Geometry check sheet. Reference: the model listing, model coordinates, mm. A direction names the side the tool comes from. Round coordinates to 2 decimals unless told otherwise and drop trailing zeros. Order: outer loops, then holes, each group sorted by start corner. A loop starts at its lowest first (then second) coordinate and runs counter-clockwise, first axis right, second up. Notation, with made-up numbers: (41, -25) -> (69, -25) arc R21 ccw to (69, 2) -> close; hole circle Ø8 at (-28.75, 2). An arc over 180 degrees is marked (long way). Use a Markdown table: item, result. Add a question column.
Item 1: Sectioned sample at A-A, the plane z = 13. Record the cut outline in (x, y).
Item 2: Sectioned sample at C-C, the plane y = 14.25. Record the cut outline in (x, z).
Item 3: Set-up check for faces 4 (the cylindrical face through (-18.66, 12.96, 23.61)), 5 (the flat face through (26.289, 10, 0)), 6 (the cylindrical face through (-4.69, 2.5, -3.59)): record each of +Z, -Z, +X, -X, +Y, -Y from which the full face is reachable in a straight line by a thin tool's end or side.
Item 4: Gauge pin test, flat ends, axial feed: pin 1 Ø6 at (x, z) = (6, 8.5) entering from +Y; pin 2 Ø6 at (x, z) = (17.907, -17.907) entering from +Y; pin 3 Ø15.5 at (x, z) = (0, 0) entering from +Y. Record the tip position at first contact, or that the pin passes through.
Item 5: Mould release check, pull along Z, two halves, no side actions. Record for faces 1 (the flat face through (0, 10, -26.289)), 2 (the flat face through (-0.4, 0, -6.2)), 3 (the cylindrical face through (15.94, 2.84, -19.71)): pulls with the +Z half, pulls with the -Z half, needs draft (parallel to the pull), parting line crosses it, or undercut.
Item 6: Material ranges on probe 1 along Z at (x, y) = (0, 3.45); probe 2 along Z at (x, y) = (-18, 16); probe 3 along Z at (x, y) = (0, 8.75), recorded low to high. Write a range as [from, to].
Item 7: Sectioned sample at B-B, the plane x = -16. Record the cut outline in (y, z), and give its area (3 significant figures).
Item 8: Sectioned sample at D-D, the plane y = 10.25. Record the cut outline in (x, z).
from build123d import *

# Parameters (mm, degrees)
SKETCH1_W       = 52.578
SKETCH1_H       = 52.578
EXTRUDE1_DEPTH  = 19.9644
EXTRUDE2_START  = -19.9644
SKETCH2_R       = 2.667
EXTRUDE2_DEPTH  = 5.7658
EXTRUDE4_START  = -19.9644
SKETCH6_R       = 5.75437
EXTRUDE4_DEPTH  = 14.1986
EXTRUDE6_START  = -45.52216
EXTRUDE6_DEPTH  = 45.52216
EXTRUDE10_START = -12.954
SKETCH15_R      = 2.8956
EXTRUDE10_DEPTH = 7.874
SKETCH16_R      = 5.9055
EXTRUDE11_DEPTH = 5.08
FILLET2_R       = 3.81
SKETCH12_R      = 5.08
EXTRUDE9_DEPTH  = 5.08


with BuildPart() as part:
    # Sketch1 → Extrude1 (new body)
    with BuildSketch(Plane(origin=(0, 0, 0), x_dir=(1, 0, 0), z_dir=(0, 1, 0))):
        Rectangle(SKETCH1_W, SKETCH1_H)
    extrude(amount=EXTRUDE1_DEPTH)

    # Sketch2 → Extrude2 (cut)
    with BuildSketch(Plane(origin=(0, 19.9644, 0), x_dir=(1, 0, 0), z_dir=(0, 1, 0)).offset(EXTRUDE2_START)):
        with Locations((-17.907, 17.907)):
            Circle(SKETCH2_R)
        with Locations((-17.907, -17.907)):
            Circle(SKETCH2_R)
        with Locations((17.907, 17.907)):
            Circle(SKETCH2_R)
    extrude(amount=EXTRUDE2_DEPTH, mode=Mode.SUBTRACT)

    # Sketch6 → Extrude4 (cut)
    with BuildSketch(Plane.XZ.offset(EXTRUDE4_START)):
        with Locations((-17.907, -17.907)):
            Circle(SKETCH6_R)
        with Locations((-17.907, 17.907)):
            Circle(SKETCH6_R)
        with Locations((17.907, -17.907)):
            Circle(SKETCH6_R)
    extrude(amount=EXTRUDE4_DEPTH, mode=Mode.SUBTRACT)

    # Sketch10 → Extrude6 (cut)
    with BuildSketch(Plane(origin=(-5.900028272, 0, -5.900028272), x_dir=(-0.707106781, 0, 0.707106781), z_dir=(-0.707106781, 0, -0.707106781)).offset(EXTRUDE6_START)):
        Polygon((-8.0645, 19.9644), (-8.0645, 17.272), (-3.6449, 12.954), (3.6449, 12.954), (8.0645, 17.272), (8.0645, 19.9644), align=None)
    extrude(amount=EXTRUDE6_DEPTH, mode=Mode.SUBTRACT)

    # Sketch15 → Extrude10 (cut)
    with BuildSketch(Plane.XZ.offset(EXTRUDE10_START)):
        Circle(SKETCH15_R)
        with Locations((11.24204, 11.24204)):
            Circle(SKETCH15_R)
    extrude(amount=EXTRUDE10_DEPTH, mode=Mode.SUBTRACT)

    # Sketch16 → Extrude11 (cut)
    with BuildSketch(Plane.XZ):
        Circle(SKETCH16_R)
        with Locations((11.24204, 11.24204)):
            Circle(SKETCH16_R)
    extrude(amount=-EXTRUDE11_DEPTH, mode=Mode.SUBTRACT)

    # Fillet2
    fillet2_edges = [part.edges().sort_by_distance(p)[0] for p in [
        (26.289, 6.477, 26.289),
        (-26.289, 9.9822, -26.289),
        (26.289, 9.9822, -26.289),
        (-26.289, 9.9822, 26.289),
    ]]
    fillet(fillet2_edges, radius=FILLET2_R)

    # Sketch12 → Extrude9 (cut)
    with BuildSketch(Plane(origin=(0, 19.9644, 0), x_dir=(1, 0, 0), z_dir=(0, 1, 0))):
        Circle(SKETCH12_R)
        with Locations((15.9004, -15.9004)):
            Circle(SKETCH12_R)
    extrude(amount=EXTRUDE9_DEPTH, mode=Mode.SUBTRACT)


solid = part.part
Found:
| question | item | result |
|---|---|---|
| 1 | outline | (-26.29, 0) -> (5.6, 0) -> (5.6, 5.08) -> (8.94, 5.08) -> (8.94, 12.95) -> (7.85, 12.95) -> (1.6, 17.27) -> (1.6, 19.96) -> (-14.9, 19.96) -> (-14.9, 5.77) -> (-20.91, 5.77) -> (-20.91, 19.96) -> (-26.29, 19.96) -> close; (13.54, 5.08) -> (16.88, 5.08) -> (16.88, 0) -> (26.29, 0) -> (26.29, 19.96) -> (24.4, 19.96) -> (24.4, 17.27) -> (18.15, 12.95) -> (13.54, 12.95) -> close |
| 2 | outline | (-26.29, -22.48) arc R3.81 ccw to (-22.48, -26.29) -> (22.48, -26.29) arc R3.81 ccw to (26.29, -22.48) -> (26.29, 19.26) -> (-2.38, -9.42) -> (-9.42, -2.38) -> (19.26, 26.29) -> (-22.48, 26.29) arc R3.81 ccw to (-26.29, 22.48) -> close; hole circle Ø11.51 at (-17.91, -17.91); hole circle Ø11.51 at (-17.91, 17.91); hole circle Ø11.51 at (17.91, -17.91) |
| 3 | face 4 | +Y |
| 3 | face 5 | +Z, -Z, +X, +Y, -Y |
| 3 | face 6 | -Y |
| 4 | pin 1 | stops at y = 14.05 |
| 4 | pin 2 | stops at y = 5.77 |
| 4 | pin 3 | stops at y = 16.96 |
| 5 | face 1 | pulls with the -Z half |
| 5 | face 2 | needs draft |
| 5 | face 3 | undercut |
| 6 | probe 1 | z = [-26.29, -5.91], [5.91, 26.29] |
| 6 | probe 2 | z = [-26.29, -23.66], [-12.15, 12.15], [23.66, 26.29] |
| 6 | probe 3 | z = [-26.29, -2.9], [2.9, 26.29] |
| 7 | outline | (0, -26.29) -> (19.96, -26.29) -> (19.96, -23.34) -> (5.77, -23.34) -> (5.77, -19.77) -> (0, -19.77) -> close; (0, -16.04) -> (5.77, -16.04) -> (5.77, -12.48) -> (19.96, -12.48) -> (19.96, 12.48) -> (5.77, 12.48) -> (5.77, 16.04) -> (0, 16.04) -> close; (0, 19.77) -> (5.77, 19.77) -> (5.77, 23.34) -> (19.96, 23.34) -> (19.96, 26.29) -> (0, 26.29) -> close |
| 7 | area | 698 mm2 |
| 8 | outline | (-26.29, -22.48) arc R3.81 ccw to (-22.48, -26.29) -> (22.48, -26.29) arc R3.81 ccw to (26.29, -22.48) -> (26.29, 22.48) arc R3.81 ccw to (22.48, 26.29) -> (-22.48, 26.29) arc R3.81 ccw to (-26.29, 22.48) -> close; hole circle Ø11.51 at (-17.91, -17.91); hole circle Ø11.51 at (-17.91, 17.91); hole circle Ø5.79 at (0, 0); hole circle Ø5.79 at (11.24, 11.24); hole circle Ø11.51 at (17.91, -17.91) |
